```python
from build123d import *

# Parameters (mm, degrees)
SKETCH_1_W      = 54
SKETCH_1_H      = 112
SKETCH_1_R      = 1.25
EXTRUDE_1_DEPTH = 1


with BuildPart() as part:
    # 草图1 → 凸台-拉伸1 (new body)
    with BuildSketch(Plane.XY):
        Rectangle(SKETCH_1_W, SKETCH_1_H)
        with Locations((-20, 16)):
            Circle(SKETCH_1_R, mode=Mode.SUBTRACT)
        with Locations((-20, -21)):
            Circle(SKETCH_1_R, mode=Mode.SUBTRACT)
        with Locations(Location((20, -21, 0), (0, 0, 180))):
            Circle(SKETCH_1_R, mode=Mode.SUBTRACT)
        with Locations(Location((20, 16, 0), (0, 0, 180))):
            Circle(SKETCH_1_R, mode=Mode.SUBTRACT)
    extrude(amount=EXTRUDE_1_DEPTH)


solid = part.part
```
Check sheet for the modelled part. Datum: model origin and axes. Units: mm. Round coordinates to 2 decimals unless told otherwise and drop trailing zeros. Order: outer loops, then holes, each group sorted by start corner. A loop starts at its lowest first (then second) coordinate and runs counter-clockwise, first axis right, second up. Notation, with made-up numbers: (74.25, 78.25) - (91.25, 78.25) arc R4 ccw to (91.25, 84.25) - close; hole circle Ø7 at (-29.75, 67.25). An arc over 180 degrees is marked (long way). Write item = value, one per line.
Q1. Draft check along X on faces 1 (the face through (-19.328, 17.054, 0.493)), 2 (the face through (0, 1, 1)). Enter one of: pulls with the +X half, pulls with the -X half, needs draft (parallel to the pull), parting line crosses it, or undercut.
Computed:
face_1 = undercut
face_2 = needs draft
Q2. Go/stop test with flat-tipped pins: pin 1 (3 mm diameter, centred on x = 20, y = -21, fed in from +Z); pin 2 (2 mm diameter, centred on x = 20, y = 16, fed in from -Z). Record where each tip stops, or that it passes through.
Computed:
pin_1 = 1
pin_2 = through
Q3. Thickness scan on line 1 along Y through (x, z) = (-20, 0.8); line 2 along Y through (x, z) = (-20.5, 0.15). Record the ranges inside material, lowest first.
Computed:
line_1 = -56 to -22.25, -19.75 to 14.75, 17.25 to 56
line_2 = -56 to -22.15, -19.85 to 14.85, 17.15 to 56
Q4. Section check A-A (x = 20). Record the boundary of the cut face in (y, z), and give its area (3 significant figures).
Computed:
outline = (-56, 0) - (-22.25, 0) - (-22.25, 1) - (-56, 1) - close; (-19.75, 0) - (14.75, 0) - (14.75, 1) - (-19.75, 1) - close; (17.25, 0) - (56, 0) - (56, 1) - (17.25, 1) - close
area = 107 mm^2
Q5. Section check B-B (y = 16). Record the boundary of the cut face in (x, z).
Computed:
outline = (-27, 0) - (-21.25, 0) - (-21.25, 1) - (-27, 1) - close; (-18.75, 0) - (18.75, 0) - (18.75, 1) - (-18.75, 1) - close; (21.25, 0) - (27, 0) - (27, 1) - (21.25, 1) - close
